from build123d import *

# Parameters (mm, degrees)
F0_W     = 32
F0_H     = 56
F1_DEPTH = 8
F2_W     = 3
F2_H     = 3
F3_DEPTH = 1
F4_W     = 24
F4_H     = 16
F5_DEPTH = 0.5
F4_W_2   = 3
F4_H_2   = 3
F4_W_3   = 2
F4_H_3   = 2
F6_DEPTH = 1
F8_DEPTH = 4.1


with BuildPart() as f1:
    # F0 (on Top) → F1 (new body)
    with BuildSketch(Plane.XY):
        Rectangle(F0_W, F0_H)
    extrude(amount=F1_DEPTH)

    # F2 (on face) → F3 (join)
    with BuildSketch(Plane.YZ.offset(16)):
        with Locations((22.5, 4)):
            Rectangle(F2_W, F2_H)
    extrude(amount=F3_DEPTH)

    # F4 (on face) → F5 (cut)
    with BuildSketch(Plane.XY.offset(8)):
        with Locations((0, 16)):
            Rectangle(F4_W, F4_H)
    extrude(amount=-F5_DEPTH, mode=Mode.SUBTRACT)

    # F4 (on face) → F6 (join)
    with BuildSketch(Plane.XY.offset(8)):
        Polygon((-10.052171, -7.5), (-13.052171, -7.5), (-13.052171, -10.5), (-10.052171, -10.5), (-10.052171, -13.5), (-7.052171, -13.5), (-7.052171, -10.5), (-4.052171, -10.5), (-4.052171, -7.5), (-7.052171, -7.5), (-7.052171, -4.5), (-10.052171, -4.5), align=None)
        with Locations((2.5, -12)):
            Rectangle(F4_W_2, F4_H_2)
        with Locations((6.5, -8)):
            Rectangle(F4_W_2, F4_H_2)
        with Locations((10.5, -4)):
            Rectangle(F4_W_2, F4_H_2)
        with Locations((-2, -21.35515)):
            Rectangle(F4_W_3, F4_H_3)
        with Locations((2, -21.35515)):
            Rectangle(F4_W_3, F4_H_3)
        Polygon((-1, -23.35515), (-2, -23.35515), (-2, -26.35515), (-1, -26.35515), (-1, -25.35515), (0, -25.35515), (1, -25.35515), (1, -26.35515), (2, -26.35515), (2, -23.35515), (1, -23.35515), (1, -22.45515), (-1, -22.45515), align=None)
    extrude(amount=F6_DEPTH)

    # F7 (on face) → F8 (cut)
    with BuildSketch(Plane.YZ.offset(16)):
        Polygon((0, 1.8), (2.192031, 3.992031), (0, 6.184062), (-2.192031, 3.992031), align=None)
    extrude(amount=-F8_DEPTH, mode=Mode.SUBTRACT)


solid = f1.part
Model file for the job. Use its own axes, mm. A direction names the side the tool comes from. Coordinates: 2 decimals unless noted, no trailing zeros. Write each loop counter-clockwise with the first axis right and the second up, starting at its lowest first coordinate (ties: lowest second). Pieces come first, ordered by that corner, then holes. Notation, with made-up numbers: (-28.75, 27) - (7.25, 27) arc R22 ccw to (7.25, 44) - close; hole circle Ø5 at (57, 89.5). An arc over 180 degrees is marked (long way). Write each question's results on one line, items separated by ' | '. Start each with the question number.
1) Mould opens along Z. For faces 4 (the face through (-11.6, -10.5, 8.5)), 5 (the face through (13.979, 1.111, 5.073)), 6 (the face through (14, 1.1, 2.9)), 7 (the face through (2, -12, 9)) say: pulls with the +Z half, pulls with the -Z half, needs draft (parallel to the pull), parting line crosses it, or undercut.
2) Cut at C-C (z = 4.75). Write the cut outline in (x, y), then the cut area to 3 significant figures.
3) 3-axis set-ups, long thin cutter, end or side, ignore diameter. For faces 1 (the face through (-10.052, -6, 8.5)), 2 (the face through (-1, -25.9, 8.5)), 3 (the face through (6.5, -9.5, 8.5)): which of +Z, -Z, +X, -X, +Y, -Y reach the whole face in a straight line?
4) Cut at A-A (y = 19.5). Write the cut outline in (x, z), then the cut area to 3 significant figures.
5) Cut at B-B (x = -11). Write the cut outline in (y, z).
6) Cut at D-D (y = -1). Write the cut outline in (x, z).
7) Flat gauge pins, fed straight in: P1, Ø0.5, axis at x = 16.5, y = 22.5, coming from the -Z side; P2, Ø0.8, axis at x = -9, z = 8.5, coming from the -Y side; P3, Ø2, axis at x = -11.5, y = 8, coming from the +Z side. Where does each tip first touch, or does it go through?
8) Probe line 1 along X through (y, z) = (-8, 8.5); line 2 along Z through (x, y) = (-10.5, 3); line 3 along X through (y, z) = (5, 7). List the from-to ranges inside material, lowest first. Write a range as from..to.
Returned:
1) face 4: needs draft | face 5: undercut | face 6: undercut | face 7: pulls with the +Z half
2) outline: (-16, -28) - (16, -28) - (16, -1.43) - (11.9, -1.43) - (11.9, 1.43) - (16, 1.43) - (16, 21) - (17, 21) - (17, 24) - (16, 24) - (16, 28) - (-16, 28) - close | area: 1,780 mm^2
3) face 1: +Z, -X, +Y | face 2: +Z, -Y | face 3: +Z, +X, -Y
4) outline: (-16, 0) - (16, 0) - (16, 8) - (12, 8) - (12, 7.5) - (-12, 7.5) - (-12, 8) - (-16, 8) - close | area: 244 mm^2
5) outline: (-28, 0) - (28, 0) - (28, 8) - (24, 8) - (24, 7.5) - (8, 7.5) - (8, 8) - (-7.5, 8) - (-7.5, 9) - (-10.5, 9) - (-10.5, 8) - (-28, 8) - close
6) outline: (-16, 0) - (16, 0) - (16, 2.8) - (11.9, 2.8) - (11.9, 5.18) - (16, 5.18) - (16, 8) - (-16, 8) - close
7) P1: z = 2.5 | P2: y = -13.5 | P3: z = 8
8) line 1: -13.05..-4.05, 5..8 | line 2: 0..8 | line 3: -16..16
